Read the model definition and answer for the solid it produces. Units are mm, in the model's axes. A direction names the side the tool comes from. Coordinates: 2 decimals unless noted, no trailing zeros. Loops run counter-clockwise (first coordinate to the right, second up) from the corner with the lowest first, then second, coordinate; pieces in that order, holes last. Notation, with made-up numbers: (-12, 23) -> (-6, 23) arc R9 ccw to (-6, 32) -> close; hole circle Ø3 at (27.5, 10). An arc over 180 degrees is marked (long way). Answer as a JSON object with one key per item and string values. Group by question number.
Q1. For faces 5 (the flat face through (0, 0, -20)), 6 (the flat face through (-17, 10, -56)), 7 (the flat face through (-15, 12, -56)), determine the directions among +Z, -Z, +X, -X, +Y, -Y from which every point of the face is accessible in a straight line to the end or side of a thin tool.
Q2. The part is cut by section C-C on y = 15.5. Write down the section's boundary in (x, z).
Q3. The part is cut by section D-D on z = 21.5. Write down the section's boundary in (x, y).
Q4. Determine the mould class of faces 1 (the cylindrical face through (27.314, 9.86, -12.408)), 2 (the flat face through (17, 10, 28)), 3 (the cylindrical face through (-27.458, 9.86, -12.086)), 4 (the cylindrical face through (0, 10, -100)) for opening direction X: released by +X, released by -X, zero draft, split by the parting line, or undercut.
Q5. The part is cut by section B-B on z = -36. Write down the section's boundary in (x, y).
Q6. Straight lines are drawn through the part: line 1 along Z through (x, y) = (0, 10.25); line 2 along X through (y, z) = (1.5, 0); line 3 along X through (y, z) = (11.75, 0). For each, find the intervals that lie inside material, in ascending order. Write a range as [from, to].
Q7. The part is cut by section A-A on x = 0. Write down the section's boundary in (y, z), and give its area (4 significant figures).
Q8. Each of these flat-tipped pins is pushed along its axis until it touches: P1, Ø1, axis at x = -14.5, y = 5, coming from the -Z side; P2, Ø8, axis at y = 3, z = -84, coming from the +X side; P3, Ø12, axis at x = 11.5, y = 10.5, coming from the -Z side. Where does it stop, or does it pass through?
Autodesk Inventor part; units mm, degrees
ref_plane "YZ Plane" through (0, 0, 0) normal (1, 0, 0) x (0, 1, 0)
ref_plane "XZ Plane" through (0, 0, 0) normal (0, 1, 0) x (-1, 0, 0)
ref_plane "XY Plane" through (0, 0, 0) normal (0, 0, 1) x (1, 0, 0)
sketch "Sketch2" plane through (0, 0, 0) normal (0, 1, 0) x (-1, 0, 0)
  circle A0 centre (0, 0) radius 30
  dimension "d0" = 60
extrude "Extrusion1" add sketch "Sketch2" along normal blind 20
sketch "Sketch3" plane through (0, 20, 0) normal (0, 1, 0) x (1, 0, 0)
  circle A0 centre (0, 0) radius 27.5
  dimension "d3" = 55
extrude "Extrusion2" cut sketch "Sketch3" against normal blind 17
sketch "Sketch4" plane through (0, 3, 0) normal (0, 1, 0) x (1, 0, 0)
  circle A0 centre (0, 0) radius 5
  dimension "d6" = 10
extrude "Extrusion3" cut sketch "Sketch4" against normal blind 5
sketch "Sketch9" plane through (0, 20, 0) normal (0, 1, 0) x (1, 0, 0)
  line L0 (-15, 35) -> (15, 35)
  line L1 (15, 35) -> (15, 20)
  line L2 (15, 20) -> (-15, 20)
  line L3 (-15, 20) -> (-15, 35)
  circle A0 centre (0, 0) radius 27.5
  line L4 (-15, 35) -> (15, 20) construction
  line L5 (15, 35) -> (-15, 20) construction
  point P0 (0, 27.5)
extrude "Extrusion6" cut sketch "Sketch9" against normal blind 17 contours L0 L1 A0 L3 | A0 L1 L2 L3 picked at (1.0554, 22.439)
sketch "Sketch10" plane through (0, 20, 0) normal (0, 1, 0) x (1, 0, 0)
  arc A0 (-15, 23.0489) -> (15, 23.0489) centre (0, 0) ccw
  line L0 (-15, 23.0489) -> (-17, 23.0489)
  line L1 (-17, 23.0489) -> (-17, 83.0489)
  line L2 (-17, 83.0489) -> (-15, 83.0489)
  line L3 (-15, 83.0489) -> (-15, 23.0489)
  line L4 (15, 25.9808) -> (15, 23.0489)
  line L5 (15, 23.0489) -> (17, 23.0489)
  line L6 (17, 23.0489) -> (17, 83.0489)
  line L7 (17, 83.0489) -> (15, 83.0489)
  line L8 (15, 83.0489) -> (15, 23.0489)
  dimension "d17" = 60
  dimension "d18" = 60
extrude "Extrusion7" add sketch "Sketch10" against normal blind 20
fillet "Fillet1" radius 13 1 edges at (-15, 11.5, -23.0489)
fillet "Fillet2" radius 9 1 edges at (-17, 10, -24.7184)
fillet "Fillet3" radius 13 1 edges at (15, 11.5, -23.0489)
fillet "Fillet4" radius 9 1 edges at (17, 10, -24.7184)
sketch "Sketch12" plane through (0, 0, 0) normal (0, -1, 0) x (1, 0, 0)
  line L0 (-15, -29.2617) -> (-15, -83.0489)
  line L1 (15, -25.9808) -> (-15, -25.9808)
  line L2 (-15, -25.9808) -> (-15, -83.0489)
  line L3 (-15, -83.0489) -> (15, -83.0489)
  line L4 (15, -83.0489) -> (15, -25.9808)
  point P0 (0, 0)
extrude "Extrusion8" add sketch "Sketch12" against normal blind 3
sketch "Sketch13" plane through (0, 20, 0) normal (0, 1, 0) x (1, 0, 0)
  arc A0 (-20, 22.3607) -> (20, 22.3607) centre (0, 0) ccw
  line L0 (30, 0) -> (28, 0)
  line L1 (28, 0) -> (28, -30)
  line L2 (28, -30) -> (30, -30)
  line L3 (30, -30) -> (30, 0)
  line L4 (-30, 0) -> (-28, 0)
  line L5 (-28, 0) -> (-28, -30)
  line L6 (-28, -30) -> (-30, -30)
  line L7 (-30, -30) -> (-30, 0)
extrude "Extrusion9" add sketch "Sketch13" against normal blind 20
sketch "Sketch14" plane through (0, 20, 0) normal (0, 1, 0) x (1, 0, 0)
  line L0 (-30, -30) -> (-30, 0)
  line L1 (30, 0) -> (30, -30)
  line L2 (-30, -30) -> (30, -30)
  line L3 (30, -30) -> (30, -28)
  line L4 (30, -28) -> (-30, -28)
  line L5 (-30, -28) -> (-30, -30)
  point P0 (0, 0)
extrude "Extrusion10" add sketch "Sketch14" against normal blind 20
sketch "Sketch17" plane through (28, 0, 10.7703) normal (-1, 0, 0) x (0, 0, 1)
  point P0 (-10.7703, 0)
sketch "Sketch21" plane through (0, 20, 0) normal (0, 1, 0) x (1, 0, 0)
  line L0 (15, 83.0489) -> (-15, 83.0489)
  line L1 (-15, 83.0489) -> (-17, 83.0489)
  arc A0 (15, 83.0489) -> (-15, 83.0489) centre (0, 82.9999) ccw
  arc A1 (17, 83.0489) -> (-17, 83.0489) centre (0, 82.9999) ccw
  line L2 (-17, 83.0489) -> (-17, 29.0689)
  line L3 (-17, 83.0489) -> (-15, 83.0489)
  line L4 (15, 83.0489) -> (17, 83.0489)
  point P0 (0, 0)
extrude "Extrusion15" add sketch "Sketch21" against normal blind 20 contours A0 L1 A1 L4
sketch "Sketch22" plane through (0, 0, 0) normal (0, -1, 0) x (1, 0, 0)
  line L0 (15, -83.0489) -> (15, -25.1247)
  arc A0 (-15, -83.0489) -> (15, -83.0489) centre (0, -82.9999) ccw
  line L1 (-15, -83.0489) -> (15, -83.0489)
  line L2 (15, -83.0489) -> (-15, -83.0489)
  point P0 (0, 0)
extrude "Extrusion16" add sketch "Sketch22" against normal blind 3
sketch "Sketch23" plane through (0, 0, 0) normal (0, -1, 0) x (1, 0, 0)
  line L0 (15.995, -25.328) -> (14.0863, -25.328)
  line L1 (14.0863, -25.328) -> (14.0863, -29.7912)
  line L2 (14.0863, -29.7912) -> (15.995, -29.7912)
  line L3 (15.995, -29.7912) -> (15.995, -25.328)
  line L4 (-13.7592, -25.328) -> (-16.454, -25.328)
  line L5 (-16.454, -25.328) -> (-16.454, -29.7912)
  line L6 (-16.454, -29.7912) -> (-13.7592, -29.7912)
  line L7 (-13.7592, -29.7912) -> (-13.7592, -25.328)
  point P0 (0, 0)
extrude "Extrusion17" add sketch "Sketch23" against normal blind 3
sketch "Sketch25" plane through (0, 20, 0) normal (0, 1, 0) x (1, 0, 0)
  line L0 (28, -28) -> (10.7703, -28)
  line L1 (28, -28) -> (21.2132, -21.2132)
  arc A0 (10.7703, -28) -> (28, -10.7703) centre (0, 0) ccw
  line L2 (28, -28) -> (37.598, -28) construction
  line L3 (28, -28) -> (23, -28)
  line L4 (23, -28) -> (18.5654, -23.5654)
  line L5 (28, -28) -> (28, -23)
  line L6 (28, -23) -> (23.5654, -18.5654)
  line L7 (23.5654, -18.5654) -> (18.5654, -23.5654)
  line L8 (21.2132, -21.2132) -> (21.0654, -21.0654)
  dimension "d53" = 135
  dimension "d54" = 5
  dimension "d55" = 135
  dimension "d56" = 5
  dimension "d57" = 135
extrude "Extrusion19" add sketch "Sketch25" against normal blind 20 contours L0 L4 A0 L1 | L1 A0 L6 L5
sketch "Sketch27" plane through (0, 20, 0) normal (0, 1, 0) x (1, 0, 0)
  line L0 (-28, -28) -> (-28, -10.7703)
  line L1 (-28, -28) -> (-21.2132, -21.2132)
  arc A0 (-28, -10.7703) -> (-10.7703, -28) centre (0, 0) ccw
  line L2 (-28, -28) -> (-18.402, -28) construction
  line L3 (-28, -28) -> (-23, -28)
  line L4 (-28, -28) -> (-28, -23)
  line L5 (-28, -23) -> (-23.5654, -18.5654)
  line L6 (-23, -28) -> (-18.5654, -23.5654)
  line L7 (-23, -28) -> (-16.7285, -28) construction
  line L8 (-18.5654, -23.5654) -> (-23.5654, -18.5654)
  dimension "d60" = 45
  dimension "d61" = 5
  dimension "d62" = 5
  dimension "d63" = 135
  dimension "d64" = 45
extrude "Extrusion20" add sketch "Sketch27" against normal blind 20 contours L0 L5 A0 L1 | L1 A0 L6 L3
properties part number "Axel chamber"
Final values:
{
 "1": {"face 5": "+Z, -Z, +X, -X, -Y", "face 6": "-Z, -X, +Y, -Y", "face 7": "+Y"},
 "2": {"outline": "(-30, 0) arc R30 ccw to (-20, -22.36) arc R9 cw to (-17, -29.07) -> (-17, -83.05) arc R17 ccw to (17, -83.05) -> (17, -29.07) arc R9 cw to (20, -22.36) arc R30 ccw to (30, 0) -> (30, 30) -> (-30, 30) -> close; hole (-28, 10.77) arc R30 cw to (-23.57, 18.57) -> (-28, 23) -> close; hole (-23, 28) -> (-18.57, 23.57) arc R30 cw to (-10.77, 28) -> close; hole (-19.01, -19.87) arc R13 cw to (-15, -29.26) -> (-15, -83.05) arc R15 ccw to (15, -83.05) -> (15, -29.26) arc R13 cw to (19.01, -19.87) arc R27.5 ccw (long way) to start; hole (10.77, 28) arc R30 cw to (18.57, 23.57) -> (23, 28) -> close; hole (23.57, 18.57) arc R30 cw to (28, 10.77) -> (28, 23) -> close"},
 "3": {"outline": "(-30, 0) -> (-28, 0) -> (-28, 20) -> (-30, 20) -> close; (-26.5, 0) -> (26.5, 0) -> (26.5, 20) -> (17.15, 20) -> (17.15, 3) -> (-17.15, 3) -> (-17.15, 20) -> (-26.5, 20) -> close; (28, 0) -> (30, 0) -> (30, 20) -> (28, 20) -> close"},
 "4": {"face 1": "released by +X", "face 2": "undercut", "face 3": "released by -X", "face 4": "split by the parting line"},
 "5": {"outline": "(-17, 0) -> (17, 0) -> (17, 20) -> (15, 20) -> (15, 3) -> (-15, 3) -> (-15, 20) -> (-17, 20) -> close"},
 "6": {"line 1": "z = [-100, -98], [27.5, 30]", "line 2": "x = [-30, -5], [5, 30]", "line 3": "x = [-30, -27.5], [27.5, 30]"},
 "7": {"outline": "(0, -100) -> (20, -100) -> (20, -98) -> (3, -98) -> (3, -5) -> (0, -5) -> close; (0, 5) -> (3, 5) -> (3, 27.5) -> (20, 27.5) -> (20, 30) -> (0, 30) -> close", "area": "436.5 mm2"},
 "8": {"P1": "stops at z = -92.64", "P2": "stops at x = 17", "P3": "stops at z = -99.09"}
}
